```python
from build123d import *

# Parameters (mm, degrees)
SKETCH_W                = 30
SKETCH_H                = 97
PAD_DEPTH               = 13
SKETCH001_W             = 30
SKETCH001_H             = 6
PAD001_DEPTH            = 15
PAD001_FACE5_W          = 30
PAD001_FACE5_H          = 6
PAD002_DEPTH            = 6
SKETCH002_W             = 28
SKETCH002_H             = 28
PAD003_DEPTH            = 30
SKETCH003_W             = 26
SKETCH003_H             = 26
PAD004_DEPTH            = 1
SKETCH004_W             = 30
SKETCH004_H             = 32
PAD005_DEPTH            = 14
SKETCH005_R             = 1.5
POCKET_DEPTH            = 10
SKETCH006_R             = 3
PAD006_DEPTH            = 85
SKETCH007_W             = 9
SKETCH007_H             = 85
POCKET001_DEPTH         = 4
SKETCH008_R             = 1.5
POCKET002_DEPTH         = 14
SKETCH028_W             = 9.5
SKETCH028_H             = 83
POCKET007_DEPTH         = 12
SKETCH029_W             = 9.5
SKETCH029_H             = 83
POCKET008_DEPTH         = 12
BODY001_PLACEMENT_ANGLE = 180


with BuildPart() as part:
    # Sketch → Pad (new body)
    with BuildSketch(Plane.XZ):
        Rectangle(SKETCH_W, SKETCH_H)
    extrude(amount=PAD_DEPTH)

    # Sketch001 (on Face6 of Pad) → Pad001 (join)
    with BuildSketch(Plane.XZ.offset(13)):
        with Locations((0, -45.5)):
            Rectangle(SKETCH001_W, SKETCH001_H)
        with Locations((0, 45.5)):
            Rectangle(SKETCH001_W, SKETCH001_H)
    extrude(amount=PAD001_DEPTH)

    # Pad001 Face5 → Pad002 (add)
    with BuildSketch(Plane(origin=(0, -28, 45.5), x_dir=(-1, 0, 0), z_dir=(0, -1, 0))):
        Rectangle(PAD001_FACE5_W, PAD001_FACE5_H)
    extrude(amount=PAD002_DEPTH)

    # Sketch002 (on Face8 of Pad002) → Pad003 (join)
    with BuildSketch(Plane(origin=(0, 0, 48.5), x_dir=(-1, 0, 0), z_dir=(0, 0, 1))):
        with Locations((0, 20)):
            Rectangle(SKETCH002_W, SKETCH002_H)
    extrude(amount=PAD003_DEPTH)

    # Sketch003 (on Face1 of Pad003) → Pad004 (join)
    with BuildSketch(Plane.XZ.offset(13)):
        with Locations((0, -19.410291)):
            Rectangle(SKETCH003_W, SKETCH003_H)
    extrude(amount=PAD004_DEPTH)

    # Sketch004 (on Face15 of Pad004) → Pad005 (join)
    with BuildSketch(Plane.XZ.offset(14)):
        with Locations((0, -19.410291)):
            Rectangle(SKETCH004_W, SKETCH004_H)
    extrude(amount=PAD005_DEPTH)

    # Sketch005 (on Face24 of Pad005) → Pocket (cut)
    with BuildSketch(Plane.XZ.offset(28)):
        with Locations((-10, -9.410291)):
            Circle(SKETCH005_R)
        with Locations((10, -9.410291)):
            Circle(SKETCH005_R)
        with Locations((10, -29.410291)):
            Circle(SKETCH005_R)
        with Locations((-10, -29.410291)):
            Circle(SKETCH005_R)
    extrude(amount=-POCKET_DEPTH, mode=Mode.SUBTRACT)

    # Sketch006 (on Face5 of Pocket) → Pad006 (join)
    with BuildSketch(Plane(origin=(0, 0, 42.5), x_dir=(1, 0, 0), z_dir=(0, 0, -1))):
        with Locations((0, 20)):
            Circle(SKETCH006_R)
    extrude(amount=PAD006_DEPTH)

    # Sketch007 (on Face1 of Pad006) → Pocket001 (cut)
    with BuildSketch(Plane.XZ.offset(13)):
        Rectangle(SKETCH007_W, SKETCH007_H)
    extrude(amount=-POCKET001_DEPTH, mode=Mode.SUBTRACT)

    # Sketch008 (on Face8 of Pocket001) → Pocket002 (cut)
    with BuildSketch(Plane(origin=(0, 0, 0), x_dir=(1, 0, 0), z_dir=(0, 1, 0))):
        with Locations((-8.5, 27.5)):
            Circle(SKETCH008_R)
        with Locations((8.5, 27.5)):
            Circle(SKETCH008_R)
        with Locations((8.5, -27.5)):
            Circle(SKETCH008_R)
        with Locations((-8.5, -27.5)):
            Circle(SKETCH008_R)
    extrude(amount=-POCKET002_DEPTH, mode=Mode.SUBTRACT)

    # Sketch028 (on Face17 of Pocket002) → Pocket007 (cut)
    with BuildSketch(Plane.XZ.offset(13)):
        with Locations((-9.25, 0)):
            Rectangle(SKETCH028_W, SKETCH028_H)
    extrude(amount=-POCKET007_DEPTH, mode=Mode.SUBTRACT)

    # Sketch029 (on Face1 of Pocket007) → Pocket008 (cut)
    with BuildSketch(Plane.XZ.offset(13)):
        with Locations((9.25, 0)):
            Rectangle(SKETCH029_W, SKETCH029_H)
    extrude(amount=-POCKET008_DEPTH, mode=Mode.SUBTRACT)


with BuildPart() as part_1:
    # Body001 placement: moved
    add(part.part.moved(Location((-1, -9, 20))).rotate(Axis((-1, -9, 20), (0, 1, 0)), BODY001_PLACEMENT_ANGLE))


solid = part_1.part
```
Read the model definition and answer for the solid it produces. Units are mm, in the model's axes. A direction names the side the tool comes from. Give positions to 0.01 mm unless a question says otherwise; leave off trailing zeros. Write each loop counter-clockwise with the first axis right and the second up, starting at its lowest first coordinate (ties: lowest second). Pieces come first, ordered by that corner, then holes. Notation, with made-up numbers: (80, -13.5) -> (84, -13.5) arc R14 ccw to (84, -3.5) -> close; hole circle Ø6 at (70, 82.5). An arc over 180 degrees is marked (long way). Answer in a Markdown table with one row per item.
1) Section A-A on z = 18 is taken. Give the vertices of the cut face in (x, y), plus the area to 3 significant figures.
Results list:
| item | result |
|---|---|
| outline | (-16, -22) -> (-15, -22) -> (-15, -10) -> (-5.5, -10) -> (-5.5, -18) -> (3.5, -18) -> (3.5, -10) -> (13, -10) -> (13, -22) -> (14, -22) -> (14, -9) -> (-16, -9) -> close; circle Ø6 at (-1, -29) |
| area | 154 mm^2 |
2) Section C-C on y = -33.5 is taken. Give the vertices of the cut face in (x, z).
Results list:
| item | result |
|---|---|
| outline | (-16, -28.5) -> (-15, -28.5) -> (-15, -58.5) -> (13, -58.5) -> (13, -28.5) -> (14, -28.5) -> (14, -22.5) -> (-16, -22.5) -> close; (-16, 23.41) -> (14, 23.41) -> (14, 55.41) -> (-16, 55.41) -> close; (-16, 62.5) -> (14, 62.5) -> (14, 68.5) -> (-16, 68.5) -> close; hole circle Ø3 at (-11, 29.41); hole circle Ø3 at (-11, 49.41); hole circle Ø3 at (9, 29.41); hole circle Ø3 at (9, 49.41) |
3) Determine the mould class of faces 5 (the flat face through (-15.4, -22, 19.8)), 6 (the flat face through (13, -29, -43)), 7 (the flat face through (-1, -22, 39)), 8 (the flat face through (-11, -27, 29)) for opening direction X: released by +X, released by -X, zero draft, split by the parting line, or undercut.
Results list:
| item | result |
|---|---|
| face 5 | zero draft |
| face 6 | released by +X |
| face 7 | undercut |
| face 8 | undercut |
4) Straight lines are drawn through the part: line 1 (Z direction, x = 7.5, y = -22.3); line 2 (Z direction, x = 1, y = -25.5); line 3 (X direction, y = -16.5, z = 20.5). For each, find the intervals that lie inside material, in ascending order. Write a range as [from, to].
Results list:
| item | result |
|---|---|
| line 1 | [-58.5, -22.5], [26.41, 46], [49, 52.41], [62.5, 68.5] |
| line 2 | [-58.5, -22.5], [23.41, 55.41], [62.5, 68.5] |
| line 3 | [-16, -15], [-5.5, 3.5], [13, 14] |
5) A tool of negligible diameter and unlimited length cuts with its end or side. For faces 1 (the flat face through (3.5, -14, 21)), 2 (the flat face through (8, -16, -21.5)), 3 (the cylindrical face through (7.825, -9.493, 46.036)), 4 (the flat face through (-15, -29, -43)), from which of +Z, -Z, +X, -X, +Y, -Y can it reach the whole face along a straight path? Write none if from no direction.
Results list:
| item | result |
|---|---|
| face 1 | none |
| face 2 | -Y |
| face 3 | +Y |
| face 4 | -Z, -X, +Y, -Y |
6) Section B-B on x = -1 is taken. Give the vertices of the cut face in (y, z), plus the area to 3 significant figures.
Results list:
| item | result |
|---|---|
| outline | (-43, -58.5) -> (-15, -58.5) -> (-15, -28.5) -> (-9, -28.5) -> (-9, 68.5) -> (-37, 68.5) -> (-37, 62.5) -> (-32, 62.5) -> (-32, 55.41) -> (-37, 55.41) -> (-37, 23.41) -> (-32, 23.41) -> (-32, -22.5) -> (-43, -22.5) -> close; hole (-26, -22.5) -> (-18, -22.5) -> (-18, 62.5) -> (-26, 62.5) -> (-26, 55.41) -> (-23, 55.41) -> (-23, 52.41) -> (-22, 52.41) -> (-22, 26.41) -> (-23, 26.41) -> (-23, 23.41) -> (-26, 23.41) -> close |
| area | 2,770 mm^2 |
7) Each of these flat-tipped pins is pushed along its axis until it touches: pin 1 Ø0.9 at (x, z) = (8.5, 29) entering from -Y; pin 2 Ø1 at (y, z) = (-33, 14.5) entering from -X; pin 3 Ø3 at (x, z) = (-2.5, 64) entering from -Y; pin 4 Ø8.5 at (y, z) = (-32.5, -43) entering from -X. Where does it stop, or does it pass through?
Results list:
| item | result |
|---|---|
| pin 1 | y = -27 |
| pin 2 | through |
| pin 3 | y = -37 |
| pin 4 | x = -15 |
8) Section D-D on z = 33 is taken. Give the vertices of the cut face in (x, y), plus the area to 3 significant figures.
Results list:
| item | result |
|---|---|
| outline | (-16, -37) -> (14, -37) -> (14, -23) -> (12, -23) -> (12, -22) -> (-14, -22) -> (-14, -23) -> (-16, -23) -> close; (-16, -22) -> (-15, -22) -> (-15, -10) -> (-5.5, -10) -> (-5.5, -18) -> (3.5, -18) -> (3.5, -10) -> (13, -10) -> (13, -22) -> (14, -22) -> (14, -9) -> (-16, -9) -> close |
| area | 572 mm^2 |
